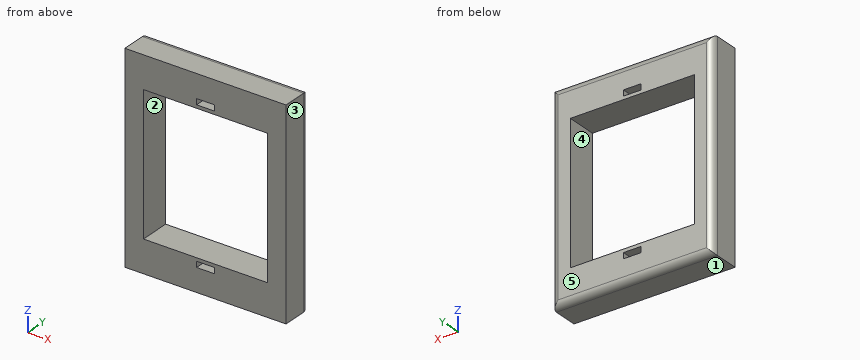
```python
from build123d import *

# Parameters (mm, degrees)
SKETCH1_W           = 50
SKETCH1_H           = 63
SKETCH1_W_2         = 38.5
SKETCH1_H_2         = 43
BOSS_EXTRUDE1_DEPTH = 9.5
SKETCH2_W           = 5.5
SKETCH2_H           = 1.8
CUT_EXTRUDE1_DEPTH  = 64.325897498
FILLET1_R           = 2


with BuildPart() as part:
    # Sketch1 → Boss-Extrude1 (new body)
    with BuildSketch(Plane(origin=(0, 0, 0), x_dir=(1, 0, 0), z_dir=(0, 1, 0))):
        with Locations((-23.459677419, 8.143145161)):
            Rectangle(SKETCH1_W, SKETCH1_H)
        with Locations((-23.459677419, 8.143145161)):
            Rectangle(SKETCH1_W_2, SKETCH1_H_2, mode=Mode.SUBTRACT)
    extrude(amount=BOSS_EXTRUDE1_DEPTH)

    # Sketch2 → Cut-Extrude1 (cut, through all)
    with BuildSketch(Plane(origin=(0, 9.5, 0), x_dir=(1, 0, 0), z_dir=(0, 1, 0))):
        with Locations((-23.459677419, 31.543145161)):
            Rectangle(SKETCH2_W, SKETCH2_H)
        with Locations((-23.459677419, -15.256854839)):
            Rectangle(SKETCH2_W, SKETCH2_H)
    extrude(amount=-CUT_EXTRUDE1_DEPTH, mode=Mode.SUBTRACT)

    # Fillet1
    fillet1_edges = [part.edges().sort_by_distance(p)[0] for p in [
        (-48.459677419, 9.5, -8.143145161),
        (-23.459677419, 9.5, 23.356854839),
        (1.540322581, 9.5, -8.143145161),
        (-23.459677419, 9.5, -39.643145161),
    ]]
    fillet(fillet1_edges, radius=FILLET1_R)


solid = part.part
```
Geometry check sheet. Reference: the model listing, model coordinates, mm. Face numbers are marked on the shaded views. A direction names the side the tool comes from. Round coordinates to 2 decimals unless told otherwise and drop trailing zeros. Order: outer loops, then holes, each group sorted by start corner. A loop starts at its lowest first (then second) coordinate and runs counter-clockwise, first axis right, second up. Notation, with made-up numbers: (56, -37.75) -> (77, -37.75) arc R21 ccw to (77, -4.75) -> close; hole circle Ø10 at (79, 38.25). An arc over 180 degrees is marked (long way). Return JSON: item names as keys, results as strings. Group by question number.
Q1. Section check A-A, the plane z = 6. Record the boundary of the cut face in (x, y), plus the area to 3 significant figures.
Q2. Section check B-B, the plane x = -23. Record the boundary of the cut face in (y, z), plus the area to 3 significant figures.
Q3. Release check for a two-part mould opening along X. For the marked faces 1, 2 and 3 record: released by +X, released by -X, zero draft, split by the parting line, or undercut.
Q4. Tool access check on the marked faces 4 and 5. Record the directions out of +Z, -Z, +X, -X, +Y, -Y that give a thin tool (end or side, any length) a straight path to the whole face; none if there is none.
Q5. Material ranges on probe 1 along Z at (x, y) = (-26, 2); probe 2 along Z at (x, y) = (-12, 0.5); probe 3 along X at (y, z) = (5, 14.5), recorded low to high. Write a range as from..to.
Q6. Section check D-D, the plane x = -14.5. Record the boundary of the cut face in (y, z).
Q7. Section check C-C, the plane y = 5.5. Record the boundary of the cut face in (x, z).
Numbers:
{
 "1": {"outline": "(-48.46, 0) -> (-42.71, 0) -> (-42.71, 9.5) -> (-46.46, 9.5) arc R2 ccw to (-48.46, 7.5) -> close; (-4.21, 0) -> (1.54, 0) -> (1.54, 7.5) arc R2 ccw to (-0.46, 9.5) -> (-4.21, 9.5) -> close", "area": "108 mm^2"},
 "2": {"outline": "(0, -39.64) -> (7.5, -39.64) arc R2 ccw to (9.5, -37.64) -> (9.5, -32.44) -> (0, -32.44) -> close; (0, -30.64) -> (9.5, -30.64) -> (9.5, -29.64) -> (0, -29.64) -> close; (0, 13.36) -> (9.5, 13.36) -> (9.5, 14.36) -> (0, 14.36) -> close; (0, 16.16) -> (9.5, 16.16) -> (9.5, 21.36) arc R2 ccw to (7.5, 23.36) -> (0, 23.36) -> close", "area": "154 mm^2"},
 "3": {"face 1": "zero draft", "face 2": "undercut", "face 3": "released by +X"},
 "4": {"face 4": "+Y, -Y", "face 5": "+Z, -Z, +X, -X, +Y"},
 "5": {"probe 1": "-39.64..-32.44, -30.64..-29.64, 13.36..14.36, 16.16..23.36", "probe 2": "-39.64..-29.64, 13.36..23.36", "probe 3": "-48.46..-26.21, -20.71..1.54"},
 "6": {"outline": "(0, -39.64) -> (7.5, -39.64) arc R2 ccw to (9.5, -37.64) -> (9.5, -29.64) -> (0, -29.64) -> close; (0, 13.36) -> (9.5, 13.36) -> (9.5, 21.36) arc R2 ccw to (7.5, 23.36) -> (0, 23.36) -> close"},
 "7": {"outline": "(-48.46, -39.64) -> (1.54, -39.64) -> (1.54, 23.36) -> (-48.46, 23.36) -> close; hole (-42.71, -29.64) -> (-4.21, -29.64) -> (-4.21, 13.36) -> (-42.71, 13.36) -> close; hole (-26.21, -32.44) -> (-20.71, -32.44) -> (-20.71, -30.64) -> (-26.21, -30.64) -> close; hole (-26.21, 14.36) -> (-20.71, 14.36) -> (-20.71, 16.16) -> (-26.21, 16.16) -> close"}
}
